Study the drawing (mm; zero at the part's minimum x, y, z) and answer. Coordinates: 2 decimals unless noted, no trailing zeros. Order: outer loops, then holes, each group sorted by start corner. A loop starts at its lowest first (then second) coordinate and runs counter-clockwise, first axis right, second up. Notation, with made-up numbers: M 14.5,19 L 57.5,19 A12 ccw 57.5,23 Z; hole C 79.5,-14 d11. An arc over 180 degrees is marked long. Put each result on its own line as item: value.
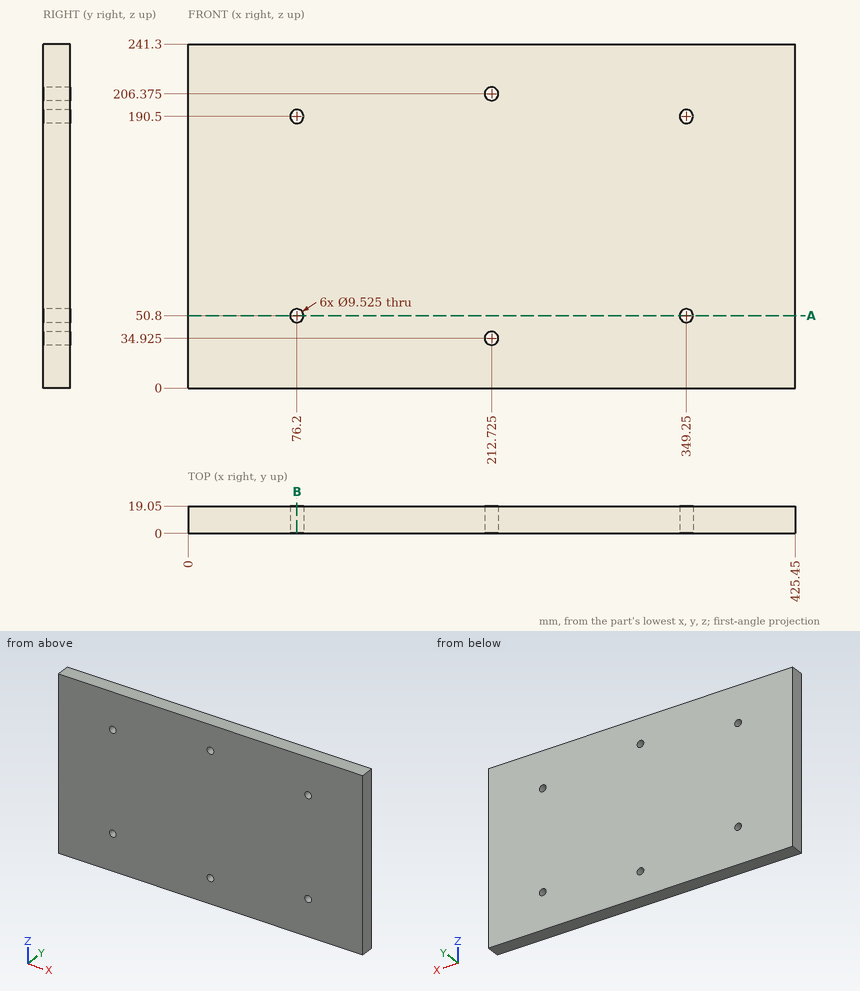
Q1. Consider line 1 along Z through (x, y) = (76.2, 12.75); line 2 along Z through (x, y) = (216, 11.25). Determine where each line is inside the solid, lowest interval first.
Answers below:
line 1: z = 0 to 46.04, 55.56 to 185.74, 195.26 to 241.3
line 2: z = 0 to 31.47, 38.38 to 202.92, 209.83 to 241.3
Q2. Find section B-B on x = 76.2. Write down the section's boundary in (y, z).
Answers below:
outline: M 0,0 L 19.05,0 L 19.05,46.04 L 0,46.04 Z; M 0,55.56 L 19.05,55.56 L 19.05,185.74 L 0,185.74 Z; M 0,195.26 L 19.05,195.26 L 19.05,241.3 L 0,241.3 Z
Q3. Find section A-A on z = 50.8. Write down the section's boundary in (x, y), plus the area to 3 significant figures.
Answers below:
outline: M 0,0 L 71.44,0 L 71.44,19.05 L 0,19.05 Z; M 80.96,0 L 344.49,0 L 344.49,19.05 L 80.96,19.05 Z; M 354.01,0 L 425.45,0 L 425.45,19.05 L 354.01,19.05 Z
area: 7,740 mm^2
